Design review of the part built by this model. Coordinates are the model's own, in mm. Face numbers are marked on the shaded views. A direction names the side the tool comes from. Coordinates: 2 decimals unless noted, no trailing zeros. Order: outer loops, then holes, each group sorted by start corner. A loop starts at its lowest first (then second) coordinate and runs counter-clockwise, first axis right, second up. Notation, with made-up numbers: (72, -6.5) -> (119, -6.5) arc R17 cw to (119, 5.5) -> close; hole circle Ø8 at (37.25, -19.5). An arc over 180 degrees is marked (long way). Use a Markdown table: item, result. Add a question column.
Q1. Wall thickness on probe 1 along Y at (x, z) = (12, 1.1); probe 2 along Z at (x, y) = (1.05, -15); probe 3 along Z at (x, y) = (0.35, -15): over which ranges is each line inside the solid? List them lowest first.
Q2. Add section C-C (y = -15). State the section outline as (x, z) points.
Q3. Insertion check: pin 1 (0.8 mm diameter, centred on x = 0.5, z = 12.5, fed in from -Y); pin 2 (0.8 mm diameter, centred on x = 0.5, z = 13.5, fed in from +Y); pin 3 (3 mm diameter, centred on x = 6.5, y = -23, fed in from +Z). Each pin has a flat end and moves straight along its axis. Give the tip position at first contact, or say it passes through.
Q4. Machinability: for the marked faces 1 and 2, which of the approach directions +Z, -Z, +X, -X, +Y, -Y give a long, thin tool a straight path to every point of the face, cutting with its end or side? Answer none if there is none.
Q5. Add section D-D (z = 18.5). State the section outline as (x, y) points.
Q6. Add section A-A (y = -9.25). State the section outline as (x, z) points.
Q7. Add section B-B (x = 13.75). State the section outline as (y, z) points, then the cut area to 3 significant figures.
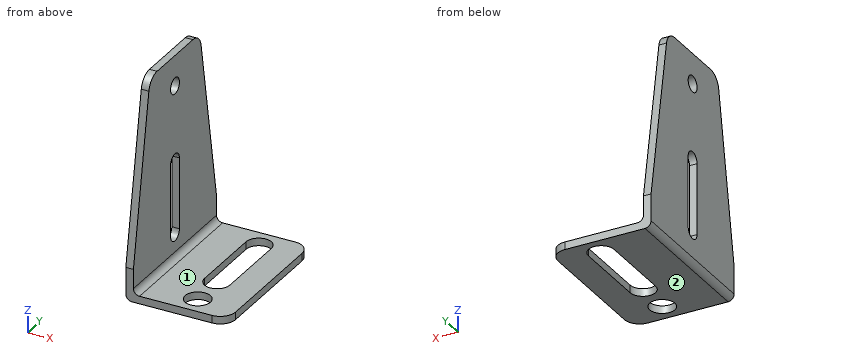
from build123d import *

# Parameters (mm, degrees)
SKETCH1_W           = 20
SKETCH1_H           = 30
SKETCH1_R           = 2.5
BOSS_EXTRUDE1_DEPTH = 1.5
SKETCH3_R           = 1.6
BOSS_EXTRUDE2_DEPTH = 1.5
FILLET1_R           = 1.2
FILLET2_R           = 3


with BuildPart() as part:
    # Sketch1 → Boss-Extrude1 (new body)
    with BuildSketch(Plane.XY):
        with Locations((10, -15)):
            Rectangle(SKETCH1_W, SKETCH1_H)
        with Locations((12, -26)):
            Circle(SKETCH1_R, mode=Mode.SUBTRACT)
        with BuildLine():
            Line((14.5, -4), (14.5, -19))
            ThreePointArc((14.5, -19), (12, -21.5), (9.5, -19))
            Line((9.5, -19), (9.5, -4))
            ThreePointArc((9.5, -4), (12, -1.5), (14.5, -4))
        make_face(mode=Mode.SUBTRACT)
    extrude(amount=BOSS_EXTRUDE1_DEPTH)

    # Sketch3 → Boss-Extrude2 (add)
    with BuildSketch(Plane.ZY):
        Polygon((1.5, 0), (1.5, -30), (6.5, -30), (41.5, -24), (41.5, -6), (6.5, 0), align=None)
        with Locations(Location((35.5, -15, 0), (0, 0, 270))):
            Circle(SKETCH3_R, mode=Mode.SUBTRACT)
        with BuildLine():
            Line((6.5, -13.4), (20.5, -13.4))
            ThreePointArc((20.5, -13.4), (22.1, -15), (20.5, -16.6))
            Line((20.5, -16.6), (6.5, -16.6))
            ThreePointArc((6.5, -16.6), (4.9, -15), (6.5, -13.4))
        make_face(mode=Mode.SUBTRACT)
    extrude(amount=-BOSS_EXTRUDE2_DEPTH)

    # Fillet1
    fillet1_edges = [part.edges().sort_by_distance(p)[0] for p in [
        (1.5, -15, 1.5),
        (0, -15, 0),
    ]]
    fillet(fillet1_edges, radius=FILLET1_R)

    # Fillet2
    fillet2_edges = [part.edges().sort_by_distance(p)[0] for p in [
        (0.75, -6, 41.5),
        (0.75, -24, 41.5),
        (20, 0, 0.75),
        (20, -30, 0.75),
    ]]
    fillet(fillet2_edges, radius=FILLET2_R)


solid = part.part
Established:
| question | item | result |
|---|---|---|
| 1 | probe 1 | -30 to -28.5, -23.5 to -21.5, -1.5 to 0 |
| 1 | probe 2 | 0.01 to 4.9, 22.1 to 33.9, 37.1 to 41.5 |
| 1 | probe 3 | 0.35 to 4.9, 22.1 to 33.9, 37.1 to 41.5 |
| 2 | outline | (0, 1.2) arc R1.2 ccw to (1.2, 0) -> (9.5, 0) -> (9.5, 1.5) -> (2.7, 1.5) arc R1.2 cw to (1.5, 2.7) -> (1.5, 4.9) -> (0, 4.9) -> close; (0, 22.1) -> (1.5, 22.1) -> (1.5, 33.9) -> (0, 33.9) -> close; (0, 37.1) -> (1.5, 37.1) -> (1.5, 41.5) -> (0, 41.5) -> close; (14.5, 0) -> (20, 0) -> (20, 1.5) -> (14.5, 1.5) -> close |
| 3 | pin 1 | y = -29.04 |
| 3 | pin 2 | y = -1.13 |
| 3 | pin 3 | z = 1.5 |
| 4 | face 1 | +Z, +X, +Y, -Y |
| 4 | face 2 | -Z, +X, -X, +Y, -Y |
| 5 | outline | (0, -27.94) -> (1.5, -27.94) -> (1.5, -16.6) -> (0, -16.6) -> close; (0, -13.4) -> (1.5, -13.4) -> (1.5, -2.06) -> (0, -2.06) -> close |
| 6 | outline | (0, 1.2) arc R1.2 ccw to (1.2, 0) -> (9.5, 0) -> (9.5, 1.5) -> (2.7, 1.5) arc R1.2 cw to (1.5, 2.7) -> (1.5, 41.5) -> (0, 41.5) -> close; (14.5, 0) -> (20, 0) -> (20, 1.5) -> (14.5, 1.5) -> close |
| 7 | outline | (-30, 0) -> (-27.79, 0) -> (-27.79, 1.5) -> (-30, 1.5) -> close; (-24.21, 0) -> (-20.79, 0) -> (-20.79, 1.5) -> (-24.21, 1.5) -> close; (-2.21, 0) -> (0, 0) -> (0, 1.5) -> (-2.21, 1.5) -> close |
| 7 | area | 11.8 mm^2 |
